Model file for the job. Use its own axes, mm. A direction names the side the tool comes from. Round coordinates to 2 decimals unless told otherwise and drop trailing zeros. Write each loop counter-clockwise with the first axis right and the second up, starting at its lowest first coordinate (ties: lowest second). Pieces come first, ordered by that corner, then holes.
```python
from build123d import *

# Parameters (mm, degrees)
SKETCH1_W            = 53
SKETCH1_H            = 153
BOSS_EXTRUDE1_DEPTH  = 3
SKETCH2_R            = 1.125
CUT_EXTRUDE1_DEPTH   = 3
SKETCH4_W            = 58
SKETCH4_H            = 3
BOSS_EXTRUDE3_DEPTH  = 4.5
SKETCH5_W            = 58
SKETCH5_H            = 3
BOSS_EXTRUDE4_DEPTH  = 4.5
SKETCH8_W            = 15
SKETCH8_H            = 13.5
CUT_EXTRUDE3_DEPTH   = 3
SKETCH9_W            = 6
SKETCH9_H            = 9
CUT_EXTRUDE4_DEPTH   = 3
SKETCH10_W           = 15
SKETCH10_H           = 10
CUT_EXTRUDE5_DEPTH   = 3
SKETCH11_W           = 12.75
SKETCH11_H           = 22.75
CUT_EXTRUDE6_DEPTH   = 3
SKETCH12_R           = 1
CUT_EXTRUDE7_DEPTH   = 3
SKETCH17_W           = 9
SKETCH17_H           = 3
BOSS_EXTRUDE6_DEPTH  = 6
SKETCH18_W           = 9
SKETCH18_H           = 3
BOSS_EXTRUDE8_DEPTH  = 6
SKETCH19_R           = 1.5
CUT_EXTRUDE11_DEPTH  = 3
SKETCH20_W           = 58
SKETCH20_H           = 3
BOSS_EXTRUDE9_DEPTH  = 6.5
SKETCH21_W           = 58
SKETCH21_H           = 3
BOSS_EXTRUDE10_DEPTH = 6.5
SKETCH29_W           = 8
SKETCH29_H           = 3
CUT_EXTRUDE15_DEPTH  = 3
SKETCH33_W           = 21
SKETCH33_H           = 17.25
CUT_EXTRUDE20_DEPTH  = 3
CHAMFER1_SIZE        = 3
CHAMFER2_SIZE        = 3
CHAMFER3_SIZE        = 3
CHAMFER4_SIZE        = 3
SKETCH34_W           = 8.25
SKETCH34_H           = 3
CUT_EXTRUDE21_DEPTH  = 3
SKETCH35_W           = 3
SKETCH35_H           = 6.75
CUT_EXTRUDE22_DEPTH  = 3
SKETCH36_W           = 3
SKETCH36_H           = 6.75
CUT_EXTRUDE23_DEPTH  = 3
SKETCH37_W           = 3
SKETCH37_H           = 10.5
CUT_EXTRUDE24_DEPTH  = 3
FILLET1_R            = 15
FILLET2_R            = 15
SKETCH38_W           = 23
SKETCH38_H           = 3
BOSS_EXTRUDE12_DEPTH = 8.25
SKETCH39_W           = 8
SKETCH39_H           = 3
CUT_EXTRUDE25_DEPTH  = 3
SKETCH40_W           = 53
SKETCH40_H           = 3
BOSS_EXTRUDE13_DEPTH = 16
SKETCH41_W           = 8
SKETCH41_H           = 3
CUT_EXTRUDE26_DEPTH  = 3
SKETCH42_R           = 8.5
SKETCH42_R_2         = 1.5
CUT_EXTRUDE30_DEPTH  = 3


with BuildPart() as part:
    # Sketch1 → Boss-Extrude1 (new body)
    with BuildSketch(Plane(origin=(0, 0, 0), x_dir=(1, 0, 0), z_dir=(0, 1, 0))):
        with Locations((13.558181818, 0)):
            Rectangle(SKETCH1_W, SKETCH1_H)
    extrude(amount=BOSS_EXTRUDE1_DEPTH)

    # Sketch2 → Cut-Extrude1 (cut)
    with BuildSketch(Plane(origin=(0, 3, 0), x_dir=(1, 0, 0), z_dir=(0, 1, 0))):
        with Locations(Location((-5.441818182, -68.25, 0), (0, 0, 270))):
            Circle(SKETCH2_R)
        with Locations(Location((-5.441818182, -51, 0), (0, 0, 270))):
            Circle(SKETCH2_R)
        with Locations(Location((32.558181818, -68.25, 0), (0, 0, 270))):
            Circle(SKETCH2_R)
        with Locations(Location((32.558181818, -51, 0), (0, 0, 270))):
            Circle(SKETCH2_R)
    extrude(amount=-CUT_EXTRUDE1_DEPTH, mode=Mode.SUBTRACT)

    # Sketch4 → Boss-Extrude3 (add)
    with BuildSketch(Plane(origin=(40.058181818, 0, 0), x_dir=(0, 0, -1), z_dir=(1, 0, 0))):
        with Locations((-2.5, 1.5)):
            Rectangle(SKETCH4_W, SKETCH4_H)
    extrude(amount=BOSS_EXTRUDE3_DEPTH)

    # Sketch5 → Boss-Extrude4 (add)
    with BuildSketch(Plane.ZY.offset(12.941818182)):
        with Locations((2.5, 1.5)):
            Rectangle(SKETCH5_W, SKETCH5_H)
    extrude(amount=BOSS_EXTRUDE4_DEPTH)

    # Sketch8 → Cut-Extrude3 (cut)
    with BuildSketch(Plane(origin=(0, 3, 0), x_dir=(1, 0, 0), z_dir=(0, 1, 0))):
        with Locations((-5.441818182, 69.75)):
            Rectangle(SKETCH8_W, SKETCH8_H)
        with Locations((32.558181818, 69.75)):
            Rectangle(SKETCH8_W, SKETCH8_H)
    extrude(amount=-CUT_EXTRUDE3_DEPTH, mode=Mode.SUBTRACT)

    # Sketch9 → Cut-Extrude4 (cut)
    with BuildSketch(Plane(origin=(0, 3, 0), x_dir=(1, 0, 0), z_dir=(0, 1, 0))):
        with Locations((-9.941818182, 58.5)):
            Rectangle(SKETCH9_W, SKETCH9_H)
        with Locations((37.058181818, 58.5)):
            Rectangle(SKETCH9_W, SKETCH9_H)
    extrude(amount=-CUT_EXTRUDE4_DEPTH, mode=Mode.SUBTRACT)

    # Sketch10 → Cut-Extrude5 (cut)
    with BuildSketch(Plane(origin=(0, 3, 0), x_dir=(1, 0, 0), z_dir=(0, 1, 0))):
        with Locations((-5.441818182, 49)):
            Rectangle(SKETCH10_W, SKETCH10_H)
        with Locations((32.558181818, 49)):
            Rectangle(SKETCH10_W, SKETCH10_H)
    extrude(amount=-CUT_EXTRUDE5_DEPTH, mode=Mode.SUBTRACT)

    # Sketch11 → Cut-Extrude6 (cut)
    with BuildSketch(Plane(origin=(0, 3, 0), x_dir=(1, 0, 0), z_dir=(0, 1, 0))):
        with Locations((13.558181818, 57.375)):
            Rectangle(SKETCH11_W, SKETCH11_H)
    extrude(amount=-CUT_EXTRUDE6_DEPTH, mode=Mode.SUBTRACT)

    # Sketch12 → Cut-Extrude7 (cut)
    with BuildSketch(Plane(origin=(0, 3, 0), x_dir=(1, 0, 0), z_dir=(0, 1, 0))):
        with Locations(Location((13.558181818, 71, 0), (0, 0, 270))):
            Circle(SKETCH12_R)
        with Locations(Location((13.558181818, 43.75, 0), (0, 0, 270))):
            Circle(SKETCH12_R)
    extrude(amount=-CUT_EXTRUDE7_DEPTH, mode=Mode.SUBTRACT)

    # Sketch17 → Boss-Extrude6 (add)
    with BuildSketch(Plane.ZY.offset(6.941818182)):
        with Locations((-58.5, 1.5)):
            Rectangle(SKETCH17_W, SKETCH17_H)
    extrude(amount=BOSS_EXTRUDE6_DEPTH)

    # Sketch18 → Boss-Extrude8 (add)
    with BuildSketch(Plane(origin=(34.058181818, 0, 0), x_dir=(0, 0, -1), z_dir=(1, 0, 0))):
        with Locations((58.5, 1.5)):
            Rectangle(SKETCH18_W, SKETCH18_H)
    extrude(amount=BOSS_EXTRUDE8_DEPTH)

    # Sketch19 → Cut-Extrude11 (cut)
    with BuildSketch(Plane(origin=(0, 3, 0), x_dir=(1, 0, 0), z_dir=(0, 1, 0))):
        with Locations(Location((35.558181818, 58.5, 0), (0, 0, 270))):
            Circle(SKETCH19_R)
        with Locations(Location((-8.441818182, 58.5, 0), (0, 0, 270))):
            Circle(SKETCH19_R)
    extrude(amount=-CUT_EXTRUDE11_DEPTH, mode=Mode.SUBTRACT)

    # Sketch20 → Boss-Extrude9 (add)
    with BuildSketch(Plane(origin=(44.558181818, 0, 0), x_dir=(0, 0, -1), z_dir=(1, 0, 0))):
        with Locations((-2.5, 1.5)):
            Rectangle(SKETCH20_W, SKETCH20_H)
    extrude(amount=BOSS_EXTRUDE9_DEPTH)

    # Sketch21 → Boss-Extrude10 (add)
    with BuildSketch(Plane.ZY.offset(17.441818182)):
        with Locations((2.5, 1.5)):
            Rectangle(SKETCH21_W, SKETCH21_H)
    extrude(amount=BOSS_EXTRUDE10_DEPTH)

    # Sketch29 → Cut-Extrude15 (cut)
    with BuildSketch(Plane(origin=(0, 3, 0), x_dir=(1, 0, 0), z_dir=(0, 1, 0))):
        with Locations((1.558181818, -49.5)):
            Rectangle(SKETCH29_W, SKETCH29_H)
        with Locations((1.558181818, -69.75)):
            Rectangle(SKETCH29_W, SKETCH29_H)
        with Locations((25.558181818, -49.5)):
            Rectangle(SKETCH29_W, SKETCH29_H)
        with Locations((25.558181818, -69.75)):
            Rectangle(SKETCH29_W, SKETCH29_H)
    extrude(amount=-CUT_EXTRUDE15_DEPTH, mode=Mode.SUBTRACT)

    # Sketch33 → Cut-Extrude20 (cut)
    with BuildSketch(Plane(origin=(0, 3, 0), x_dir=(1, 0, 0), z_dir=(0, 1, 0))):
        with Locations((13.558181818, -59.625)):
            Rectangle(SKETCH33_W, SKETCH33_H)
    extrude(amount=-CUT_EXTRUDE20_DEPTH, mode=Mode.SUBTRACT)

    # Chamfer1
    chamfer1_edges = [part.edges().sort_by_distance(p)[0] for p in [
        (-12.941818182, 1.5, -54),
    ]]
    chamfer(chamfer1_edges, length=CHAMFER1_SIZE)

    # Chamfer2
    chamfer2_edges = [part.edges().sort_by_distance(p)[0] for p in [
        (-12.941818182, 1.5, -63),
    ]]
    chamfer(chamfer2_edges, length=CHAMFER2_SIZE)

    # Chamfer3
    chamfer3_edges = [part.edges().sort_by_distance(p)[0] for p in [
        (40.058181818, 1.5, -54),
    ]]
    chamfer(chamfer3_edges, length=CHAMFER3_SIZE)

    # Chamfer4
    chamfer4_edges = [part.edges().sort_by_distance(p)[0] for p in [
        (40.058181818, 1.5, -63),
    ]]
    chamfer(chamfer4_edges, length=CHAMFER4_SIZE)

    # Sketch34 → Cut-Extrude21 (cut)
    with BuildSketch(Plane(origin=(0, 3, 0), x_dir=(1, 0, 0), z_dir=(0, 1, 0))):
        with Locations((-15.691818182, 25)):
            Rectangle(SKETCH34_W, SKETCH34_H)
        with Locations((42.808181818, 25)):
            Rectangle(SKETCH34_W, SKETCH34_H)
        with Locations((-15.691818182, -30)):
            Rectangle(SKETCH34_W, SKETCH34_H)
        with Locations((42.808181818, -30)):
            Rectangle(SKETCH34_W, SKETCH34_H)
        with Locations((13.558181818, -30)):
            Rectangle(SKETCH34_W, SKETCH34_H)
        with Locations((13.558181818, 25)):
            Rectangle(SKETCH34_W, SKETCH34_H)
    extrude(amount=-CUT_EXTRUDE21_DEPTH, mode=Mode.SUBTRACT)

    # Sketch35 → Cut-Extrude22 (cut)
    with BuildSketch(Plane(origin=(0, 3, 0), x_dir=(1, 0, 0), z_dir=(0, 1, 0))):
        with Locations((42.808181818, 16.75)):
            Rectangle(SKETCH35_W, SKETCH35_H)
        with Locations((42.808181818, -21.75)):
            Rectangle(SKETCH35_W, SKETCH35_H)
    extrude(amount=-CUT_EXTRUDE22_DEPTH, mode=Mode.SUBTRACT)

    # Sketch36 → Cut-Extrude23 (cut)
    with BuildSketch(Plane(origin=(0, 3, 0), x_dir=(1, 0, 0), z_dir=(0, 1, 0))):
        with Locations((13.474653765, 16.75)):
            Rectangle(SKETCH36_W, SKETCH36_H)
        with Locations((13.474653765, -21.75)):
            Rectangle(SKETCH36_W, SKETCH36_H)
    extrude(amount=-CUT_EXTRUDE23_DEPTH, mode=Mode.SUBTRACT)

    # Sketch37 → Cut-Extrude24 (cut)
    with BuildSketch(Plane(origin=(0, 3, 0), x_dir=(1, 0, 0), z_dir=(0, 1, 0))):
        with Locations((-20.441818182, 13)):
            Rectangle(SKETCH37_W, SKETCH37_H)
        with Locations((-20.441818182, -18)):
            Rectangle(SKETCH37_W, SKETCH37_H)
    extrude(amount=-CUT_EXTRUDE24_DEPTH, mode=Mode.SUBTRACT)

    # Fillet1
    fillet1_edges = [part.edges().sort_by_distance(p)[0] for p in [
        (-12.941818182, 1.5, -44),
    ]]
    fillet(fillet1_edges, radius=FILLET1_R - 0.0001)  # a hair under: the kernel refuses the full size

    # Fillet2
    fillet2_edges = [part.edges().sort_by_distance(p)[0] for p in [
        (40.058181818, 1.5, -44),
    ]]
    fillet(fillet2_edges, radius=FILLET2_R - 0.0001)  # a hair under: the kernel refuses the full size

    # Sketch38 → Boss-Extrude12 (add)
    with BuildSketch(Plane(origin=(0, 0, -76.5), x_dir=(-1, 0, 0), z_dir=(0, 0, -1))):
        with Locations((-13.558181818, 1.5)):
            Rectangle(SKETCH38_W, SKETCH38_H)
    extrude(amount=BOSS_EXTRUDE12_DEPTH)

    # Sketch39 → Cut-Extrude25 (cut)
    with BuildSketch(Plane(origin=(0, 0, 0), x_dir=(-1, 0, 0), z_dir=(0, -1, 0))):
        with Locations((-8.308181818, 81.75)):
            Rectangle(SKETCH39_W, SKETCH39_H)
        with Locations((-18.808181818, 81.75)):
            Rectangle(SKETCH39_W, SKETCH39_H)
    extrude(amount=-CUT_EXTRUDE25_DEPTH, mode=Mode.SUBTRACT)

    # Sketch40 → Boss-Extrude13 (add)
    with BuildSketch(Plane.XY.offset(76.5)):
        with Locations((13.558181818, 1.5)):
            Rectangle(SKETCH40_W, SKETCH40_H)
    extrude(amount=BOSS_EXTRUDE13_DEPTH)

    # Sketch41 → Cut-Extrude26 (cut)
    with BuildSketch(Plane(origin=(0, 3, 0), x_dir=(1, 0, 0), z_dir=(0, 1, 0))):
        with Locations((-6.691818182, -89.5)):
            Rectangle(SKETCH41_W, SKETCH41_H)
        with Locations((33.808181818, -89.5)):
            Rectangle(SKETCH41_W, SKETCH41_H)
        with Locations((13.558181818, -89.5)):
            Rectangle(SKETCH41_W, SKETCH41_H)
    extrude(amount=-CUT_EXTRUDE26_DEPTH, mode=Mode.SUBTRACT)

    # Sketch42 → Cut-Extrude30 (cut)
    with BuildSketch(Plane(origin=(0, 3, 0), x_dir=(1, 0, 0), z_dir=(0, 1, 0))):
        with Locations(Location((13.558181818, -2.5, 0), (0, 0, 270))):
            Circle(SKETCH42_R)
        with Locations(Location((30.558181818, 14.5, 0), (0, 0, 270))):
            Circle(SKETCH42_R_2)
        with Locations(Location((-3.441818182, 14.5, 0), (0, 0, 270))):
            Circle(SKETCH42_R_2)
        with Locations(Location((-3.441818182, -19.5, 0), (0, 0, 270))):
            Circle(SKETCH42_R_2)
        with Locations(Location((30.558181818, -19.5, 0), (0, 0, 270))):
            Circle(SKETCH42_R_2)
        Polygon((8.058181818, 14.75), (8.058181818, 11.194345135), (19.058181818, 11.194345135), (19.058181818, 14.75), (26.058181818, 14.75), (26.058181818, 7.75), (1.058181818, 7.75), (1.058181818, 14.75), align=None)
    extrude(amount=-CUT_EXTRUDE30_DEPTH, mode=Mode.SUBTRACT)


solid = part.part
```
1) Wall check: probe 1 along Z at (x, y) = (44, 2.2) (3 decimals); probe 2 along Z at (x, y) = (-20, 0.7); probe 3 along X at (y, z) = (2.85, -24.5). Give the ranges that are in metal, low to high.
2) Which spindle directions (+Z, -Z, +X, -X, +Y, -Y) get a long thin tool onto all of the face, cutting with end or side? Do faces 5 (the face through (-22, 1, -26.5)), 6 (the face through (-19.817, 2, 30)), 7 (the face through (-11.567, 2, -25)). Say none if no direction does.
3) Pull direction X, two halves, no side cores. Call faces 1 (the face through (40.058, 2, -58)), 2 (the face through (-12.942, 1, 62)), 3 (the face through (-11.567, 2, 30)), 4 (the face through (-4, 1, -63)): released by +X, released by -X, zero draft, split by the parting line, or undercut.
4) Cut at B-B on y = 1.4. Give the number of separate pieces and of enclosed holes in the cut face, and give its area (3 significant figures).
5) Cut at A-A on z = 59. List the corners of the cut face in (x, y).
6) Flat gauge pins, fed straight in: pin 1 Ø1.6 at (x, z) = (13.56, -43.75) entering from -Y; pin 2 Ø12 at (x, z) = (11.5, -30) entering from -Y; pin 3 Ø1.5 at (y, z) = (1, 48.5) entering from +X; pin 4 Ø1.1 at (x, y) = (39.5, 2) entering from -Z. Where does each tip first touch, or does it go through?
Result sheet:
1. probe 1: z = -23.5 to -20.125, -13.375 to 18.375, 25.125 to 28.5
1. probe 2: z = -26.5 to -18.25, -7.75 to 12.75, 23.25 to 31.5
1. probe 3: x = -23.94 to -19.82, -11.57 to 9.43, 17.68 to 38.68, 46.93 to 51.06
2. face 5: -Z, -X, +Y, -Y
2. face 6: +Z, +Y, -Y
2. face 7: +Y, -Y
3. face 1: released by +X
3. face 2: released by -X
3. face 3: undercut
3. face 4: zero draft
4. separate pieces: 1
4. enclosed holes: 29
4. area: 8,010 mm2
5. outline: (-12.94, 0) - (3.06, 0) - (3.06, 3) - (-12.94, 3) - close; (24.06, 0) - (40.06, 0) - (40.06, 3) - (24.06, 3) - close
6. pin 1: passes through
6. pin 2: stops at y = 0
6. pin 3: stops at x = 40.06
6. pin 4: stops at z = -61.11
